```python
from build123d import *

# Parameters (mm, degrees)
SKETCH_1_R      = 14.5
SKETCH_1_R_2    = 0.7
EXTRUDE_1_DEPTH = 1


with BuildPart() as part:
    # 草图1 → 凸台-拉伸1 (new body)
    with BuildSketch(Plane(origin=(0, 0, 0), x_dir=(0, 0, -1), z_dir=(1, 0, 0))):
        with BuildLine():
            Line((-3.211317774, 18.212288109), (-3.820259909, 21.665770566))
            Line((-3.820259909, 21.665770566), (-0.820259909, 21.665770566))
            Line((-0.820259909, 21.665770566), (-0.820259909, 17.726539554))
            Line((-0.820259909, 17.726539554), (0.820259909, 17.726539554))
            Line((0.820259909, 17.726539554), (0.820259909, 21.665770566))
            Line((0.820259909, 21.665770566), (3.820259909, 21.665770566))
            Line((3.820259909, 21.665770566), (3.211317774, 18.212288109))
            ThreePointArc((3.211317774, 18.212288109), (3.290307164, 17.84423731), (3.603621065, 17.635586614))
            ThreePointArc((3.603621065, 17.635586614), (0, -18), (-3.603621065, 17.635586614))
            ThreePointArc((-3.603621065, 17.635586614), (-3.290307164, 17.84423731), (-3.211317774, 18.212288109))
        make_face()
        Circle(SKETCH_1_R, mode=Mode.SUBTRACT)
        with Locations((-2.1, 20)):
            Circle(SKETCH_1_R_2, mode=Mode.SUBTRACT)
        with Locations(Location((2.1, 20, 0), (0, 0, 180))):
            Circle(SKETCH_1_R_2, mode=Mode.SUBTRACT)
    extrude(amount=EXTRUDE_1_DEPTH)


solid = part.part
```
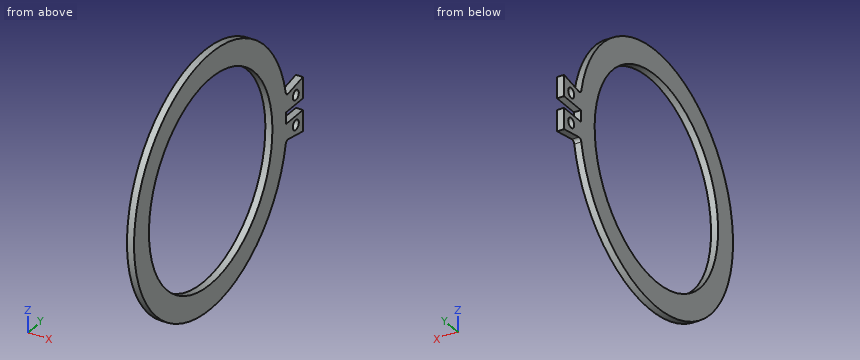
Geometry check sheet. Reference: the model listing, model coordinates, mm. Coordinates: 2 decimals unless noted, no trailing zeros. Order: outer loops, then holes, each group sorted by start corner. A loop starts at its lowest first (then second) coordinate and runs counter-clockwise, first axis right, second up. Notation, with made-up numbers: (-34.75, -6) - (-6.75, -6) arc R14 cw to (-6.75, 3) - close; hole circle Ø6 at (57, -24.5). An arc over 180 degrees is marked (long way). Answer as a JSON object with one key per item and string values. Group by question number.
Item 1: Sectioned sample at D-D, the plane z = -9.5. Record the cut outline in (x, y).
Item 2: Sectioned sample at B-B, the plane x = 0.2. Record the cut outline in (y, z), and give its area (3 significant figures).
Item 3: Scan lines: probe 1 along Z at (x, y) = (0.55, -0.5); probe 2 along Y at (x, z) = (0.2, 2.1); probe 3 along Y at (x, z) = (0.2, 6). Record each from-to range of solid material in increasing order.
Item 4: Depth check by flat-ended pin: pin 1 Ø1.8 at (y, z) = (20, -2.1) entering from -X; pin 2 Ø0.8 at (y, z) = (20, 2.1) entering from -X; pin 3 Ø0.5 at (x, y) = (0.5, 19) entering from -Z. Enter the tip coordinate at first touch or a pass-through.
Item 5: Sectioned sample at C-C, the plane z = -2.1. Record the cut outline in (x, y).
Item 6: Sectioned sample at A-A, the plane y = 0. Record the cut outline in (x, z).
Resolved:
{
 "1": {"outline": "(0, -15.29) - (1, -15.29) - (1, -10.95) - (0, -10.95) - close; (0, 10.95) - (1, 10.95) - (1, 15.29) - (0, 15.29) - close"},
 "2": {"outline": "(17.64, -3.6) arc R0.5 cw to (18.21, -3.21) - (21.67, -3.82) - (21.67, -0.82) - (17.73, -0.82) - (17.73, 0.82) - (21.67, 0.82) - (21.67, 3.82) - (18.21, 3.21) arc R0.5 cw to (17.64, 3.6) arc R18 ccw (long way) to start; hole circle Ø29 at (0, 0); hole circle Ø1.4 at (20, -2.1); hole circle Ø1.4 at (20, 2.1)", "area": "374 mm^2"},
 "3": {"probe 1": "-17.99 to -14.49, 14.49 to 17.99", "probe 2": "-17.88 to -14.35, 14.35 to 19.3, 20.7 to 21.67", "probe 3": "-16.97 to -13.2, 13.2 to 16.97"},
 "4": {"pin 1": "x = 0", "pin 2": "through", "pin 3": "z = -3.39"},
 "5": {"outline": "(0, -17.88) - (1, -17.88) - (1, -14.35) - (0, -14.35) - close; (0, 14.35) - (1, 14.35) - (1, 19.3) - (0, 19.3) - close; (0, 20.7) - (1, 20.7) - (1, 21.67) - (0, 21.67) - close"},
 "6": {"outline": "(0, -18) - (1, -18) - (1, -14.5) - (0, -14.5) - close; (0, 14.5) - (1, 14.5) - (1, 18) - (0, 18) - close"}
}
